from build123d import *

# Parameters (mm, degrees)
SKETCH1_W           = 101.6
SKETCH1_H           = 76.2
BOSS_EXTRUDE1_DEPTH = 38.1


with BuildPart() as part:
    # Sketch1 → Boss-Extrude1 (new body)
    with BuildSketch(Plane.XY):
        Polygon((0, 0), (101.6, 114.3), (127, 114.3), (127, 88.9), (177.8, 88.9), (177.8, 114.3), (228.6, 114.3), (228.6, 88.9), (279.4, 88.9), (279.4, 114.3), (304.8, 114.3), (406.4, 0), (304.8, -114.3), (279.4, -114.3), (279.4, -88.9), (228.6, -88.9), (228.6, -114.3), (177.8, -114.3), (177.8, -88.9), (127, -88.9), (127, -114.3), (101.6, -114.3), align=None)
        with Locations((126.483076325, 0)):
            Rectangle(SKETCH1_W, SKETCH1_H, mode=Mode.SUBTRACT)
        with Locations((279.4, 0)):
            Rectangle(SKETCH1_W, SKETCH1_H, mode=Mode.SUBTRACT)
    extrude(amount=BOSS_EXTRUDE1_DEPTH)


solid = part.part
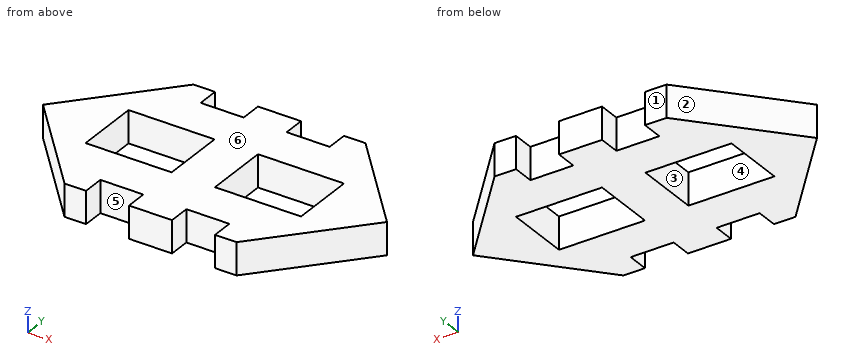
For this review, take the finished solid that the model builds, in its own axes (mm). Face numbers are marked on the shaded views. A direction names the side the tool comes from. Give positions to 0.01 mm unless a question says otherwise; leave off trailing zeros. Loops run counter-clockwise (first coordinate to the right, second up) from the corner with the lowest first, then second, coordinate; pieces in that order, holes last.
Item 1: Draft analysis for pull direction X (two halves, no side actions). For the marked faces 1, 2 and 3, state which applies: +X half, -X half, draft (parallel to the pull), parting line (faces both ways), or undercut.
Item 2: Take a section at D-D, the plane y = 12.5. State the section outline as (x, z) points.
Item 3: Tool access review of the marked faces 4, 5 and 6: name each direction out of +Z, -Z, +X, -X, +Y, -Y from which nothing blocks a thin tool from reaching the whole face with its end or side.
Item 4: Take a section at A-A, the plane y = -18. State the section outline as (x, z) points, and give its area (3 significant figures).
Item 5: For line 1 along Y through (x, z) = (247.5, 32); line 2 along Y through (x, z) = (299, 22); line 3 along X through (y, z) = (97.5, 12), list the stretches that pass through material, from the lowest coordinate up.
Item 6: Take a section at B-B, the plane z = 34. Give the number of separate pieces and of enclosed holes in the cut face, and give its area (3 significant figures).
Item 7: Insertion check: pin 1 (12.5 mm diameter, centred on y = -101, z = 20.5, fed in from -X); pin 2 (7.5 mm diameter, centred on y = 104.5, z = 21, fed in from +X); pin 3 (12 mm diameter, centred on y = -78, z = 22.5, fed in from +X). Each pin has a flat end and moves straight along its axis. Give the tip position at first contact, or say it passes through.
Item 8: Take a section at C-C, the plane x = 285.5. State the section outline as (y, z) points, and give its area (3 significant figures).
Calculated:
1. face 1: draft
1. face 2: -X half
1. face 3: undercut
2. outline: (11.11, 0) - (75.68, 0) - (75.68, 38.1) - (11.11, 38.1) - close; (177.28, 0) - (228.6, 0) - (228.6, 38.1) - (177.28, 38.1) - close; (330.2, 0) - (395.29, 0) - (395.29, 38.1) - (330.2, 38.1) - close
3. face 4: +Z, -Z
3. face 5: +Z, -Z, -Y
3. face 6: +Z, +X, -X, +Y, -Y
4. outline: (16, 0) - (75.68, 0) - (75.68, 38.1) - (16, 38.1) - close; (177.28, 0) - (228.6, 0) - (228.6, 38.1) - (177.28, 38.1) - close; (330.2, 0) - (390.4, 0) - (390.4, 38.1) - (330.2, 38.1) - close
4. area: 6,520 mm2
5. line 1: y = -88.9 to -38.1, 38.1 to 88.9
5. line 2: y = -114.3 to -38.1, 38.1 to 114.3
5. line 3: x = 86.67 to 127, 177.8 to 228.6, 279.4 to 319.73
6. separate pieces: 1
6. enclosed holes: 2
6. area: 49,000 mm2
7. pin 1: stops at x = 84.22
7. pin 2: stops at x = 316.84
7. pin 3: stops at x = 342.4
8. outline: (-114.3, 0) - (-38.1, 0) - (-38.1, 38.1) - (-114.3, 38.1) - close; (38.1, 0) - (114.3, 0) - (114.3, 38.1) - (38.1, 38.1) - close
8. area: 5,810 mm2
